```python
from build123d import *

# Parameters (mm, degrees)
SKETCH1_W           = 254.5
SKETCH1_H           = 172
BOSS_EXTRUDE1_DEPTH = 1
SKETCH2_W           = 230
SKETCH2_H           = 148
BOSS_EXTRUDE2_DEPTH = 9
SKETCH3_R           = 1.75
CUT_EXTRUDE1_DEPTH  = 2


with BuildPart() as part:
    # Sketch1 → Boss-Extrude1 (new body)
    with BuildSketch(Plane.XY):
        Rectangle(SKETCH1_W, SKETCH1_H)
    extrude(amount=BOSS_EXTRUDE1_DEPTH)

    # Sketch2 → Boss-Extrude2 (add)
    with BuildSketch(Plane(origin=(0, 0, 0), x_dir=(-1, 0, 0), z_dir=(0, 0, -1))):
        with Locations((0, -2.5)):
            Rectangle(SKETCH2_W, SKETCH2_H)
    extrude(amount=BOSS_EXTRUDE2_DEPTH)

    # Sketch3 → Cut-Extrude1 (cut)
    with BuildSketch(Plane(origin=(0, 0, -9), x_dir=(-1, 0, 0), z_dir=(0, 0, -1))):
        with Locations((29, -26.5)):
            Circle(SKETCH3_R)
        with Locations((-29, -26.5)):
            Circle(SKETCH3_R)
        with Locations((-29, 22.5)):
            Circle(SKETCH3_R)
        with Locations((29, 22.5)):
            Circle(SKETCH3_R)
    extrude(amount=-CUT_EXTRUDE1_DEPTH, mode=Mode.SUBTRACT)


solid = part.part
```
Check sheet for the modelled part. Datum: model origin and axes. Units: mm. A direction names the side the tool comes from. Give positions to 0.01 mm unless a question says otherwise; leave off trailing zeros. Write each loop counter-clockwise with the first axis right and the second up, starting at its lowest first coordinate (ties: lowest second). Pieces come first, ordered by that corner, then holes. Notation, with made-up numbers: (80.25, -33.5) - (132.25, -33.5) arc R18 cw to (132.25, -20.5) - close; hole circle Ø10 at (-37, 75.5). An arc over 180 degrees is marked (long way). Answer as a JSON object with one key per item and string values. Group by question number.
1) Access from +Z, -Z, +X, -X, +Y, -Y to the whole of each face (thin tool, end or side, straight path). Record for faces 1 (the face through (2, 71.5, -4)), 2 (the face through (115, -4, -4)), 3 (the face through (-115, -4, -4)), 4 (the face through (2, -1, -9)), 5 (the face through (2, -76.5, -4)).
2) Sectioned sample at B-B (y = -65.5). Record the cut outline in (x, z), then the cut area to 3 significant figures.
3) Depth check by flat-ended pin: P1, Ø1, axis at x = 44, z = -3, coming from the +Y side; P2, Ø3, axis at y = -62, z = -3, coming from the +X side; P3, Ø3, axis at x = -29, y = 22.5, coming from the -Z side. Enter the tip coordinate at first touch or a pass-through.
4) Sectioned sample at A-A (x = -109). Record the cut outline in (y, z), then the cut area to 3 significant figures.
5) Sectioned sample at C-C (z = -2.75). Record the cut outline in (x, y).
6) Thickness scan on probe 1 along Y at (x, z) = (-29, -7.8); probe 2 along X at (y, z) = (-18.5, -3.5); probe 3 along Y at (x, z) = (46, -3.75). Record the ranges inside material, lowest first. Write a range as from..to.
Geometry results:
{
 "1": {"face 1": "-Z, +X, -X, +Y", "face 2": "-Z, +X, +Y, -Y", "face 3": "-Z, -X, +Y, -Y", "face 4": "-Z, +X, -X, +Y, -Y", "face 5": "-Z, +X, -X, -Y"},
 "2": {"outline": "(-127.25, 0) - (-115, 0) - (-115, -9) - (115, -9) - (115, 0) - (127.25, 0) - (127.25, 1) - (-127.25, 1) - close", "area": "2,320 mm^2"},
 "3": {"P1": "stops at y = 71.5", "P2": "stops at x = 115", "P3": "stops at z = -7"},
 "4": {"outline": "(-86, 0) - (-76.5, 0) - (-76.5, -9) - (71.5, -9) - (71.5, 0) - (86, 0) - (86, 1) - (-86, 1) - close", "area": "1,500 mm^2"},
 "5": {"outline": "(-115, -76.5) - (115, -76.5) - (115, 71.5) - (-115, 71.5) - close"},
 "6": {"probe 1": "y = -76.5..-28.25, -24.75..20.75, 24.25..71.5", "probe 2": "x = -115..115", "probe 3": "y = -76.5..71.5"}
}
